```python
from build123d import *

# Parameters (mm, degrees)
F4_SIZE = 0.762


with BuildPart() as f1:
    # F0 (on Top) → F1 (revolve)
    with BuildSketch(Plane.XY):
        Polygon((0, -25.4), (2.5, -25.4), (2.5, -22.6676009336), (0, -24.1109766066), align=None)
        Polygon((2.5, -22.6676009336), (2.5, -25.4), (6.2352499547, -25.4), (6.2352499547, -24.9117339176), (5.08, -24.2447500453), (5.08, -1.1552499547), (6.2352499547, -0.4882660824), (6.2352499547, 0), (2.5, 0), align=None)
    revolve(axis=Axis((0, -12.0554883033, 0), (0, 1, 0)))

    # F2 (on face) → F3 (join, up to the next surface of F1)
    with BuildSketch(Plane(origin=(0, 0, 0), x_dir=(-1, 0, 0), z_dir=(0, 1, 0))):
        with BuildLine():
            ThreePointArc((1.570660689, 1.945), (0, 2.5), (-1.570660689, 1.945))
            Line((-1.570660689, 1.945), (1.570660689, 1.945))
        make_face()
    extrude(until=Until.NEXT, dir=(0, -1, 0))

    # F4
    f4_edges = [f1.edges().sort_by_distance(p)[0] for p in [
        (0, 0, -2.5),
        (0, 0, 1.945),
    ]]
    chamfer(f4_edges, length=F4_SIZE)


solid = f1.part
```
Check sheet for the modelled part. Datum: model origin and axes. Units: mm. A direction names the side the tool comes from. Coordinates: 2 decimals unless noted, no trailing zeros. Write each question's results on one line, items separated by ' | '. Start each with the question number.
1) Draft check along Y on faces 3 (the face through (0, -25.4, 0)), 4 (the face through (-0.05, -23.88, -0.4)), 5 (the face through (-0.661, -12.538, -5.037)). Enter one of: pulls with the +Y half, pulls with the -Y half, needs draft (parallel to the pull), parting line crosses it, or undercut.
2) Depth check by flat-ended pin: pin 1 (4 mm diameter, centred on y = -8.5, z = 3, fed in from +X); pin 2 (4 mm diameter, centred on x = 2.5, y = -18.5, fed in from +Z); pin 3 (1.6 mm diameter, centred on x = -0.5, y = -12.5, fed in from -Z). Enter the tip coordinate at first touch or a pass-through.
3) Material ranges on line 1 along Z through (x, y) = (0, -8.5) (3 decimals); line 2 along X through (y, z) = (-12.5, 0); line 3 along Y through (x, z) = (1.75, 5), recorded low to high.
4) Set-up check for faces 1 (the face through (0, -12, 1.945)), 2 (the face through (5.76, -25.15, 2.39)): record each of +Z, -Z, +X, -X, +Y, -Y from which the full face is reachable in a straight line by a thin tool's end or side.
Checked values:
1) face 3: pulls with the -Y half | face 4: pulls with the +Y half | face 5: undercut
2) pin 1: x = 4.98 | pin 2: z = 5.06 | pin 3: z = -5.08
3) line 1: -5.08 to -2.5, 1.945 to 5.08 | line 2: -5.08 to -2.5, 2.5 to 5.08 | line 3: -25.4 to -24.37, -1.03 to 0
4) face 1: +Y | face 2: +Y, -Y
